Geometry check sheet. Reference: the model listing, model coordinates, mm. A direction names the side the tool comes from. Coordinates: 2 decimals unless noted, no trailing zeros. Order: outer loops, then holes, each group sorted by start corner. A loop starts at its lowest first (then second) coordinate and runs counter-clockwise, first axis right, second up. Notation, with made-up numbers: M 51.5,-19.75 L 65.5,-19.75 A19 ccw 65.5,-5.75 Z; hole C -3.5,54 d10. An arc over 180 degrees is marked long. Use CSV: the item, a comma, the result in double quotes. Start each with the question number.
```python
from build123d import *

# Parameters (mm, degrees)
PAD_DEPTH       = 125
PAD001_DEPTH    = 3
POCKET_DEPTH    = 17
POCKET001_DEPTH = 17
POCKET002_DEPTH = 20


with BuildPart() as part:
    # Sketch → Pad (new body)
    with BuildSketch(Plane.XY):
        with BuildLine():
            ThreePointArc((15, 32.726136), (0, 35.9999996561), (-15, 32.726136))
            Line((-15, 32.726136), (-15, 36))
            ThreePointArc((-7.5, 38.272052), (-11.3072125351, 37.3248834793), (-15, 36))
            Line((-7.5, 38.272052), (-4, 43))
            Line((-4, 43), (4, 43))
            Line((7.5, 38.272052), (4, 43))
            ThreePointArc((15, 36), (11.3072125351, 37.3248834793), (7.5, 38.272052))
            Line((15, 32.726136), (15, 36))
        make_face()
    extrude(amount=PAD_DEPTH)

    # Sketch003 → Pad001 (join)
    with BuildSketch(Plane.XY):
        with BuildLine():
            ThreePointArc((-15, 4.999998377), (0, -10), (15, 4.999998377))
            Line((15, 4.999998377), (15.000003, 32.7261349689))
            ThreePointArc((15.000003, 32.7261349689), (0, 36), (-15.000003, 32.7261349689))
            Line((-15.000003, 32.7261349689), (-15, 4.999998377))
        make_face()
    extrude(amount=PAD001_DEPTH)

    # Sketch004 → Pocket (cut)
    with BuildSketch(Plane.XY.offset(111)):
        with BuildLine():
            ThreePointArc((15, 32.726136), (0, 35.9999996561), (-15, 32.726136))
            Line((-15, 32.726136), (-15, 36))
            ThreePointArc((15, 36), (0, 38.9999999735), (-15, 36))
            Line((15, 32.726136), (15, 36))
        make_face()
    extrude(amount=-POCKET_DEPTH, mode=Mode.SUBTRACT)

    # Sketch005 → Pocket001 (cut)
    with BuildSketch(Plane.XY.offset(46)):
        with BuildLine():
            ThreePointArc((15, 32.726136), (0, 35.9999996561), (-15, 32.726136))
            Line((-15, 32.726136), (-15, 36))
            ThreePointArc((15, 36), (0, 38.9999999735), (-15, 36))
            Line((15, 32.726136), (15, 36))
        make_face()
    extrude(amount=-POCKET001_DEPTH, mode=Mode.SUBTRACT)

    # Sketch006 → Pocket002 (cut)
    with BuildSketch(Plane.XZ.offset(-35)):
        with BuildLine():
            ThreePointArc((3, 104), (0, 107), (-3, 104))
            Line((-3, 104), (-3, 101))
            ThreePointArc((-3, 101), (0, 98), (3, 101))
            Line((3, 101), (3, 104))
        make_face()
        with BuildLine():
            ThreePointArc((3, 39), (0, 42), (-3, 39))
            Line((-3, 39), (-3, 36))
            ThreePointArc((-3, 36), (0, 33), (3, 36))
            Line((3, 36), (3, 39))
        make_face()
    extrude(amount=-POCKET002_DEPTH, mode=Mode.SUBTRACT)


solid = part.part
```
1) Material ranges on line 1 along Z through (x, y) = (-10.5, 37); line 2 along Z through (x, y) = (3.5, 32); line 3 along Y through (x, z) = (5.5, 7), recorded low to high.
2) Set-up check for faces 1 (the face through (3.455, 38.847, 37.619)), 2 (the face through (3, 41, 37)), 3 (the face through (0, 36, 70)): record each of +Z, -Z, +X, -X, +Y, -Y from which the full face is reachable in a straight line by a thin tool's end or side.
3) Section check C-C on y = 28.5. Record the boundary of the cut face in (x, z).
4) Section check B-B on z = 91. Record the boundary of the cut face in (x, y).
5) Gauge pin test, flat ends, axial feed: P1, Ø3.5, axis at y = 40, z = 103, coming from the -X side; P2, Ø1, axis at x = -5, z = 51, coming from the +Y side; P3, Ø2.5, axis at y = 41, z = 102.5, coming from the +X side. Record the tip position at first contact, or that the pin passes through.
6) Section check A-A on x = 0. Record the boundary of the cut face in (y, z).
7) Draft check along X on faces 4 (the face through (11.36, 37.31, 69.66)), 5 (the face through (0, 38, 125)), 6 (the face through (3.455, 38.847, 102.619)), 7 (the face through (-11.255, 37.341, 69.664)). Enter one of: +X half, -X half, draft (parallel to the pull), parting line (faces both ways), or undercut.
8) Section check D-D on y = -1. Record the boundary of the cut face in (x, z), then the cut area to 3 significant figures.
Results are:
1,line 1,"z = 0 to 29, 46 to 94, 111 to 125"
1,line 2,"z = 0 to 3"
1,line 3,"y = 35.58 to 40.97"
2,face 1,"-Y"
2,face 2,"+Y, -Y"
2,face 3,"+Z, -Y"
3,outline,"M -15,0 L 15,0 L 15,3 L -15,3 Z"
4,outline,"M -15,32.73 A36 cw 15,32.73 L 15,36 A39 ccw 7.5,38.27 L 4,43 L -4,43 L -7.5,38.27 A39 ccw -15,36 Z"
5,P1,"stops at x = -7.5"
5,P2,"stops at y = 42.32"
5,P3,"stops at x = 6.41"
6,outline,"M -10,0 L 43,0 L 43,33 L 39,33 L 39,29 L 36,29 L 36,3 L -10,3 Z; M 36,46 L 39,46 L 39,42 L 43,42 L 43,98 L 39,98 L 39,94 L 36,94 Z; M 36,111 L 39,111 L 39,107 L 43,107 L 43,125 L 36,125 Z"
7,face 4,"+X half"
7,face 5,"draft"
7,face 6,"undercut"
7,face 7,"-X half"
8,outline,"M -13.75,0 L 13.75,0 L 13.75,3 L -13.75,3 Z"
8,area,"82.5 mm²"
